The listing builds one solid part. Answer for the finished solid, in the listing's coordinates (mm). A direction names the side the tool comes from. Give positions to 0.01 mm unless a question says otherwise; leave off trailing zeros. Order: outer loops, then holes, each group sorted by start corner. A loop starts at its lowest first (then second) coordinate and runs counter-clockwise, first axis right, second up.
```python
from build123d import *

# Parameters (mm, degrees)
F1_DEPTH = 50
F3_DEPTH = 50
F4_W     = 3.671517
F4_H     = 3
F4_W_2   = 6.401138
F5_DEPTH = 50


with BuildPart() as f1:
    # F0 (on Top) → F1 (new body)
    with BuildSketch(Plane.XY):
        Polygon((18.104074, -17.248757), (18.104074, 17.248757), (15.104074, 17.248757), (1.519567, 5.748757), (1.519567, 2.748757), (-1.480433, 2.748757), (-1.480433, 5.748757), (-15.104074, 17.248757), (-18.104074, 17.248757), (-18.104074, -17.248757), align=None)
    extrude(amount=F1_DEPTH)

    # F2 (on Top) → F3 (cut)
    with BuildSketch(Plane.XY):
        Polygon((6.1, -10.048757), (-6.1, -10.048757), (-6.1, -13.048757), (-3.1, -13.048757), (-3.1, -21.213451), (3.1, -21.213451), (3.1, -13.048757), (6.1, -13.048757), align=None)
    extrude(amount=F3_DEPTH, mode=Mode.SUBTRACT)

    # F4 (on Top) → F5 (cut)
    with BuildSketch(Plane.XY):
        with Locations((-16.939832, 1.248757)):
            Rectangle(F4_W, F4_H)
        with Locations((18.304643, 1.248757)):
            Rectangle(F4_W_2, F4_H)
    extrude(amount=F5_DEPTH, mode=Mode.SUBTRACT)


solid = f1.part
```
1) For a pull along Y with two mould halves and no side action, classify faces 1 (the flat face through (-3.1, -15, 25)), 2 (the flat face through (-5, -13.049, 25)), 3 (the flat face through (10, -17.249, 25)), 4 (the flat face through (-6.1, -12, 25)) as +Y half, -Y half, draft (parallel to the pull), parting line (faces both ways), or undercut.
Geometry says:
face 1: draft
face 2: undercut
face 3: -Y half
face 4: undercut
2) Find section A-A (y = -11). Write down the section's boundary in (x, z), then the cut area to 3 significant figures.
Geometry says:
outline: (-18.1, 0) - (-6.1, 0) - (-6.1, 50) - (-18.1, 50) - close; (6.1, 0) - (18.1, 0) - (18.1, 50) - (6.1, 50) - close
area: 1,200 mm2
3) Given P1, Ø3.5, axis at x = -0.5, z = 17, coming from the +Y side; P2, Ø2, axis at x = 13.5, z = 39, coming from the +Y side; P3, Ø3.5, axis at x = 4.5, z = 24, coming from the +Y side, each flat-ended and moving along its own axis, determine where each tip first touches the part or whether it passes through.
Geometry says:
P1: stops at y = 6.4
P2: stops at y = 16.74
P3: stops at y = 9.75
4) Find section C-C (x = -5). Write down the section's boundary in (y, z), then the cut area to 3 significant figures.
Geometry says:
outline: (-17.25, 0) - (-13.05, 0) - (-13.05, 50) - (-17.25, 50) - close; (-10.05, 0) - (8.72, 0) - (8.72, 50) - (-10.05, 50) - close
area: 1,150 mm2
5) A tool of negligible diameter and unlimited length cuts with its end or side. For faces 5 (the flat face through (18.104, 10, 25)), 6 (the flat face through (17, -0.251, 25)), 7 (the flat face through (8.41, 11.58, 24.65)), 8 (the flat face through (0, -10.049, 25)), 9 (the flat face through (-15.104, 1, 25)), from which of +Z, -Z, +X, -X, +Y, -Y can it reach the whole face along a straight path? Write none if from no direction.
Geometry says:
face 5: +Z, -Z, +X, +Y, -Y
face 6: +Z, -Z, +X
face 7: +Z, -Z, +Y
face 8: +Z, -Z
face 9: +Z, -Z, -X
6) Straight lines are drawn through the part: probe 1 along X at (y, z) = (-14, 37); probe 2 along X at (y, z) = (5.5, 6); probe 3 along X at (y, z) = (1.5, 2). For each, find the intervals that lie inside material, in ascending order.
Geometry says:
probe 1: x = -18.1 to -3.1, 3.1 to 18.1
probe 2: x = -18.1 to -1.48, 1.52 to 18.1
probe 3: x = -15.1 to 15.1
7) Find section B-B (z = 7.5). Write down the section's boundary in (x, y).
Geometry says:
outline: (-18.1, -17.25) - (-3.1, -17.25) - (-3.1, -13.05) - (-6.1, -13.05) - (-6.1, -10.05) - (6.1, -10.05) - (6.1, -13.05) - (3.1, -13.05) - (3.1, -17.25) - (18.1, -17.25) - (18.1, -0.25) - (15.1, -0.25) - (15.1, 2.75) - (18.1, 2.75) - (18.1, 17.25) - (15.1, 17.25) - (1.52, 5.75) - (1.52, 2.75) - (-1.48, 2.75) - (-1.48, 5.75) - (-15.1, 17.25) - (-18.1, 17.25) - (-18.1, 2.75) - (-15.1, 2.75) - (-15.1, -0.25) - (-18.1, -0.25) - close
8) Find section D-D (y = 0.5). Write down the section's boundary in (x, z), then the cut area to 3 significant figures.
Geometry says:
outline: (-15.1, 0) - (15.1, 0) - (15.1, 50) - (-15.1, 50) - close
area: 1,510 mm2
